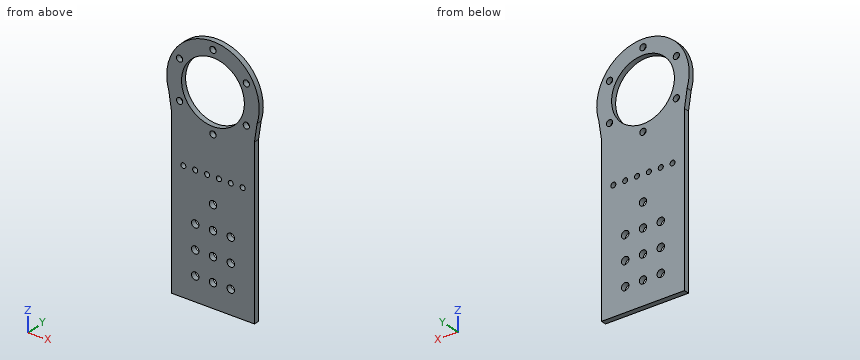
```python
from build123d import *

# Parameters (mm, degrees)
SKETCH1_R               = 39
SKETCH1_R_2             = 26.5
BOSS_EXTRUDE1_DEPTH     = 2.25
SKETCH3_W               = 50
SKETCH3_H               = 51.5
BOSS_EXTRUDE2_DEPTH     = 2.25
BOSS_EXTRUDE4_DEPTH     = 2.25
SKETCH2_R               = 2.625
CUT_EXTRUDE1_DEPTH      = 3.25
CIRPATTERN1_COUNT       = 6
CUT_EXTRUDE3_START      = -5.5
SKETCH7_R               = 3.125
CUT_EXTRUDE3_DEPTH      = 6.5
LPATTERN3_COUNT         = 3
LPATTERN3_PITCH         = 20
SKETCH8_R               = 3.125
CUT_EXTRUDE4_DEPTH      = 10
LPATTERN4_COUNT         = 4
LPATTERN4_PITCH         = 20
CUT_EXTRUDE5_START      = -5.5
SKETCH9_R               = 2.125
CUT_EXTRUDE5_DEPTH      = 6.5
LPATTERN5_COUNT         = 3
LPATTERN5_PITCH         = 10
MIRROR1_START           = -5.5
MIRROR1_COPY_1_SKETCH_R = 2.125
MIRROR1_COPY_1_DEPTH    = 6.5
MIRROR1_COPY_2_SKETCH_R = 2.125
MIRROR1_COPY_2_DEPTH    = 6.5


with BuildPart() as part:
    # Sketch1 → Boss-Extrude1 (new body, symmetric)
    with BuildSketch(Plane(origin=(0, 0, 0), x_dir=(1, 0, 0), z_dir=(0, 1, 0))):
        Circle(SKETCH1_R)
        Circle(SKETCH1_R_2, mode=Mode.SUBTRACT)
    extrude(amount=BOSS_EXTRUDE1_DEPTH, both=True)

    # Sketch3 → Boss-Extrude2 (add, symmetric)
    with BuildSketch(Plane(origin=(0, 0, 0), x_dir=(1, 0, 0), z_dir=(0, 1, 0))):
        with Locations((0, 52.25)):
            Rectangle(SKETCH3_W, SKETCH3_H)
    extrude(amount=BOSS_EXTRUDE2_DEPTH, both=True)

    # Sketch6 → Boss-Extrude4 (add, symmetric)
    with BuildSketch(Plane(origin=(0, 0, 0), x_dir=(1, 0, 0), z_dir=(0, 1, 0))):
        Polygon((-35, 166.5), (-35, 26.5), (-39, 0), (-14.981514186, 26.5), (16.520833333, 26.5), (39, 0), (35, 26.5), (35, 166.5), align=None)
    extrude(amount=BOSS_EXTRUDE4_DEPTH, both=True)

    # Sketch2 → Cut-Extrude1 (cut, symmetric)
    with BuildSketch(Plane(origin=(0, 0, 0), x_dir=(1, 0, 0), z_dir=(0, 1, 0))):
        with Locations((0, 32.5)):
            Circle(SKETCH2_R)
    cut_extrude1 = extrude(amount=CUT_EXTRUDE1_DEPTH, both=True, mode=Mode.SUBTRACT)

    # CirPattern1: Cut-Extrude1 ×6 about axis
    cirpattern1_axis = Axis((0, 0, 0), (0, 1, 0))
    for i in range(1, CIRPATTERN1_COUNT):
        add(cut_extrude1.rotate(cirpattern1_axis, i * 360 / CIRPATTERN1_COUNT), mode=Mode.SUBTRACT)

    # Sketch7 → Cut-Extrude3 (cut)
    with BuildSketch(Plane(origin=(0, 2.25, 0), x_dir=(1, 0, 0), z_dir=(0, 1, 0)).offset(CUT_EXTRUDE3_START)):
        with Locations((-15, 146.5)):
            Circle(SKETCH7_R)
        with Locations((15, 146.5)):
            Circle(SKETCH7_R)
    cut_extrude3 = extrude(amount=CUT_EXTRUDE3_DEPTH, mode=Mode.SUBTRACT)

    # LPattern3: Cut-Extrude3 ×3
    with Locations(*[(0, 0, i * LPATTERN3_PITCH) for i in range(1, LPATTERN3_COUNT)]):
        add(cut_extrude3, mode=Mode.SUBTRACT)

    # Sketch8 → Cut-Extrude4 (cut)
    with BuildSketch(Plane(origin=(0, 2.25, 0), x_dir=(1, 0, 0), z_dir=(0, 1, 0))):
        with Locations((0, 146.5)):
            Circle(SKETCH8_R)
    cut_extrude4 = extrude(amount=-CUT_EXTRUDE4_DEPTH, mode=Mode.SUBTRACT)

    # LPattern4: Cut-Extrude4 ×4
    with Locations(*[(0, 0, i * LPATTERN4_PITCH) for i in range(1, LPATTERN4_COUNT)]):
        add(cut_extrude4, mode=Mode.SUBTRACT)

    # Sketch9 → Cut-Extrude5 (cut)
    with BuildSketch(Plane(origin=(0, 2.25, 0), x_dir=(1, 0, 0), z_dir=(0, 1, 0)).offset(CUT_EXTRUDE5_START)):
        with Locations((25, 65)):
            Circle(SKETCH9_R)
    cut_extrude5 = extrude(amount=CUT_EXTRUDE5_DEPTH, mode=Mode.SUBTRACT)

    # LPattern5: Cut-Extrude5 ×3
    with Locations(*[(-i * LPATTERN5_PITCH, 0, 0) for i in range(1, LPATTERN5_COUNT)]):
        add(cut_extrude5, mode=Mode.SUBTRACT)

    # Mirror1: Cut-Extrude5 across plane
    add(cut_extrude5.mirror(Plane(origin=(0, 0, 0), x_dir=(0, 0, 1), z_dir=(1, 0, 0))), mode=Mode.SUBTRACT)

    # Mirror1 copy 1 sketch → Mirror1 copy 1 (cut)
    with BuildSketch(Plane(origin=(10, 2.25, 0), x_dir=(-1, 0, 0), z_dir=(0, 1, 0)).offset(MIRROR1_START)):
        with Locations((25, -65)):
            Circle(MIRROR1_COPY_1_SKETCH_R)
    extrude(amount=MIRROR1_COPY_1_DEPTH, mode=Mode.SUBTRACT)

    # Mirror1 copy 2 sketch → Mirror1 copy 2 (cut)
    with BuildSketch(Plane(origin=(20, 2.25, 0), x_dir=(-1, 0, 0), z_dir=(0, 1, 0)).offset(MIRROR1_START)):
        with Locations((25, -65)):
            Circle(MIRROR1_COPY_2_SKETCH_R)
    extrude(amount=MIRROR1_COPY_2_DEPTH, mode=Mode.SUBTRACT)


solid = part.part
```
Geometry: final body of the model. Coordinates: model frame, mm. Coordinates: 2 decimals unless noted, no trailing zeros. Write each loop counter-clockwise with the first axis right and the second up, starting at its lowest first coordinate (ties: lowest second). Pieces come first, ordered by that corner, then holes. Notation, with made-up numbers: M 10,82.25 L 46,82.25 A14 ccw 46,96.25 Z; hole C -9.75,56.25 d8. An arc over 180 degrees is marked long. Answer as CSV lines item,"result". Start each with the question number.
Q1. Cut plane A-A on z = -86.5. Return the cut outline in (x, y) (3 decimals).
Q2. Cut plane C-C on z = -65. Return the cut outline in (x, y) (3 decimals), then the cut area to 3 significant figures.
Q3. Line query: line 1 (Z direction, x = 28, y = -0.8); line 2 (Z direction, x = -12.5, y = 0.55) (3 decimals); line 3 (X direction, y = 0, z = -16.25). Output: solid intervals per line, ascending. Write a range as from..to.
Q4. Cut plane B-B on x = -5. Return the cut outline in (y, z) (3 decimals).
Q5. Pin query (flat end, axial travel): P1, Ø1.5, axis at y = 1.5, z = -33, coming from the -X side. Return the tip coordinate at first contact, or that it passes through.
Q6. Cut plane D-D on x = -15. Return the cut outline in (y, z) (3 decimals), then the cut area to 3 significant figures.
Findings below:
1,outline,"M -35,-2.25 L -3.125,-2.25 L -3.125,2.25 L -35,2.25 Z; M 3.125,-2.25 L 35,-2.25 L 35,2.25 L 3.125,2.25 Z"
2,outline,"M -35,-2.25 L -27.125,-2.25 L -27.125,2.25 L -35,2.25 Z; M -22.875,-2.25 L -17.125,-2.25 L -17.125,2.25 L -22.875,2.25 Z; M -12.875,-2.25 L -7.125,-2.25 L -7.125,2.25 L -12.875,2.25 Z; M -2.875,-2.25 L 2.875,-2.25 L 2.875,2.25 L -2.875,2.25 Z; M 7.125,-2.25 L 12.875,-2.25 L 12.875,2.25 L 7.125,2.25 Z; M 17.125,-2.25 L 22.875,-2.25 L 22.875,2.25 L 17.125,2.25 Z; M 27.125,-2.25 L 35,-2.25 L 35,2.25 L 27.125,2.25 Z"
2,area,"200 mm2"
3,line 1,"z = -166.5..-18.87, -13.63..13.63, 18.87..27.15"
3,line 2,"z = -166.5..-148.375, -144.625..-128.375, -124.625..-108.375, -104.625..-23.367, 23.367..36.943"
3,line 3,"x = -36.55..-30.77, -25.52..-20.93, 20.93..25.52, 30.77..36.55"
4,outline,"M -2.25,-166.5 L 2.25,-166.5 L 2.25,-67.125 L -2.25,-67.125 Z; M -2.25,-62.875 L 2.25,-62.875 L 2.25,-26.024 L -2.25,-26.024 Z; M -2.25,26.024 L 2.25,26.024 L 2.25,38.678 L -2.25,38.678 Z"
5,P1,"stops at x = -35"
6,outline,"M -2.25,-166.5 L 2.25,-166.5 L 2.25,-149.625 L -2.25,-149.625 Z; M -2.25,-143.375 L 2.25,-143.375 L 2.25,-129.625 L -2.25,-129.625 Z; M -2.25,-123.375 L 2.25,-123.375 L 2.25,-109.625 L -2.25,-109.625 Z; M -2.25,-103.375 L 2.25,-103.375 L 2.25,-67.125 L -2.25,-67.125 Z; M -2.25,-62.875 L 2.25,-62.875 L 2.25,-21.846 L -2.25,-21.846 Z; M -2.25,21.846 L 2.25,21.846 L 2.25,36 L -2.25,36 Z"
6,area,"611 mm2"
